Build history of the part. All positions in model axes, mm. Round coordinates to 2 decimals unless told otherwise and drop trailing zeros. Order: outer loops, then holes, each group sorted by start corner. A loop starts at its lowest first (then second) coordinate and runs counter-clockwise, first axis right, second up. Notation, with made-up numbers: (12.5, 77.25) -> (67.5, 77.25) arc R34 ccw to (67.5, 114.25) -> close; hole circle Ø8 at (43, 73.5). An arc over 180 degrees is marked (long way). Answer as CSV lines item,"result". Start each with the question number.
Autodesk Inventor part; units mm, degrees
ref_plane "YZ Plane" through (0, 0, 0) normal (1, 0, 0) x (0, 1, 0)
ref_plane "XZ Plane" through (0, 0, 0) normal (0, 1, 0) x (-1, 0, 0)
ref_plane "XY Plane" through (0, 0, 0) normal (0, 0, 1) x (1, 0, 0)
sketch "Sketch1" plane through (0, 0, 0) normal (0, 1, 0) x (-1, 0, 0)
  circle A0 centre (0, 0) radius 1.5
  line L0 (-2.5, -1.4434) -> (-2.5, 1.4434)
  line L1 (-2.5, 1.4434) -> (0, 2.8868)
  line L2 (0, 2.8868) -> (2.5, 1.4434)
  line L3 (2.5, 1.4434) -> (2.5, -1.4434)
  line L4 (2.5, -1.4434) -> (0, -2.8868)
  line L5 (0, -2.8868) -> (-2.5, -1.4434)
  point P0 (-2.5, 0)
  dimension "d0" = 3
  dimension "d1" = 5
extrude "Extrusion1" add sketch "Sketch1" along normal blind 30
properties part number "Varrilla_Cobre"
Q1. Slice it at A-A, the plane z = 0. Write the cut outline in (x, y).
Q2. Slice it at B-B, the plane y = 21.25. Write the cut outline in (x, z).
Q3. Slice it at D-D, the plane z = -1.15. Write the cut outline in (x, y).
Q4. Slice it at C-C, the plane x = 1.9. Write the cut outline in (y, z).
Q5. Probe L1, parallel to X at y = 13.5, z = -0.35; L2, parallel to Z at x = 0.9, y = 9; L3, parallel to X at y = 15.25, z = -1. List the from-to ranges inside material, lowest first.
Q6. Two-plate mould, pull along X, no slides. Class faces 1 (the face through (1.5, 14.79, -0.07)), 2 (the face through (1.15, 0, -1.24)), 3 (the face through (-1.267, 14.79, -2.155)): +X half, -X half, draft (parallel to the pull), parting line (faces both ways), or undercut.
Solutions:
1,outline,"(-2.5, 0) -> (-1.5, 0) -> (-1.5, 30) -> (-2.5, 30) -> close; (1.5, 0) -> (2.5, 0) -> (2.5, 30) -> (1.5, 30) -> close"
2,outline,"(-2.5, -1.44) -> (0, -2.89) -> (2.5, -1.44) -> (2.5, 1.44) -> (0, 2.89) -> (-2.5, 1.44) -> close; hole circle Ø3 at (0, 0)"
3,outline,"(-2.5, 0) -> (-0.96, 0) -> (-0.96, 30) -> (-2.5, 30) -> close; (0.96, 0) -> (2.5, 0) -> (2.5, 30) -> (0.96, 30) -> close"
4,outline,"(0, -1.79) -> (30, -1.79) -> (30, 1.79) -> (0, 1.79) -> close"
5,L1,"x = -2.5 to -1.46, 1.46 to 2.5"
5,L2,"z = -2.37 to -1.2, 1.2 to 2.37"
5,L3,"x = -2.5 to -1.12, 1.12 to 2.5"
6,face 1,"undercut"
6,face 2,"draft"
6,face 3,"-X half"
